from build123d import *

# Parameters (mm, degrees)
SKETCH1_R           = 1.5
SKETCH1_R_2         = 11.43
BOSS_EXTRUDE1_DEPTH = 7.62
CUT_EXTRUDE1_DEPTH  = 5.08
BOSS_EXTRUDE2_DEPTH = 2.54
SKETCH4_R           = 1
CUT_EXTRUDE2_DEPTH  = 8.62


with BuildPart() as part:
    # Sketch1 → Boss-Extrude1 (new body)
    with BuildSketch(Plane(origin=(0, 0, 0), x_dir=(1, 0, 0), z_dir=(0, 1, 0))):
        with BuildLine():
            Line((6.35, 0), (44.45, 0))
            ThreePointArc((44.45, 0), (48.940128061, 1.859871939), (50.8, 6.35))
            Line((50.8, 6.35), (50.8, 44.45))
            ThreePointArc((50.8, 44.45), (48.940128061, 48.940128061), (44.45, 50.8))
            Line((44.45, 50.8), (6.35, 50.8))
            ThreePointArc((6.35, 50.8), (1.859871939, 48.940128061), (0, 44.45))
            Line((0, 44.45), (0, 6.35))
            ThreePointArc((0, 6.35), (1.859871939, 1.859871939), (6.35, 0))
        make_face()
        with Locations((6.35, 6.35)):
            Circle(SKETCH1_R, mode=Mode.SUBTRACT)
        with Locations((6.35, 44.45)):
            Circle(SKETCH1_R, mode=Mode.SUBTRACT)
        with Locations((44.45, 44.45)):
            Circle(SKETCH1_R, mode=Mode.SUBTRACT)
        with Locations((44.45, 6.35)):
            Circle(SKETCH1_R, mode=Mode.SUBTRACT)
        with Locations((25.4, 25.4)):
            Circle(SKETCH1_R_2, mode=Mode.SUBTRACT)
    extrude(amount=BOSS_EXTRUDE1_DEPTH)

    # Sketch2 → Cut-Extrude1 (cut)
    with BuildSketch(Plane.XZ):
        with BuildLine():
            Line((8.938918626, -26.67), (0, -26.67))
            Line((0, -26.67), (0, -50.8))
            Line((0, -50.8), (24.13, -50.8))
            Line((24.13, -50.8), (24.13, -41.861081374))
            ThreePointArc((24.13, -41.861081374), (13.725667043, -37.074332957), (8.938918626, -26.67))
        make_face()
        with BuildLine():
            Line((0, 0), (0, -24.13))
            Line((0, -24.13), (8.938918626, -24.13))
            ThreePointArc((8.938918626, -24.13), (13.725667043, -13.725667043), (24.13, -8.938918626))
            Line((24.13, -8.938918626), (24.13, 0))
            Line((24.13, 0), (0, 0))
        make_face()
        with BuildLine():
            ThreePointArc((41.861081374, -26.67), (37.074332957, -37.074332957), (26.67, -41.861081374))
            Line((26.67, -41.861081374), (26.67, -50.8))
            Line((26.67, -50.8), (50.8, -50.8))
            Line((50.8, -50.8), (50.8, -26.67))
            Line((50.8, -26.67), (41.861081374, -26.67))
        make_face()
        with BuildLine():
            Line((26.67, 0), (26.67, -8.938918626))
            ThreePointArc((26.67, -8.938918626), (37.074332957, -13.725667043), (41.861081374, -24.13))
            Line((41.861081374, -24.13), (50.8, -24.13))
            Line((50.8, -24.13), (50.8, 0))
            Line((50.8, 0), (26.67, 0))
        make_face()
    extrude(amount=-CUT_EXTRUDE1_DEPTH, mode=Mode.SUBTRACT)

    # Sketch3 → Boss-Extrude2 (add)
    with BuildSketch(Plane(origin=(0, 7.62, 0), x_dir=(1, 0, 0), z_dir=(0, 1, 0))):
        with BuildLine():
            Line((35.63906734, 20.32), (15.16093266, 20.32))
            ThreePointArc((15.16093266, 20.32), (25.4, 13.97), (35.63906734, 20.32))
        make_face()
        with BuildLine():
            ThreePointArc((15.16093266, 30.48), (13.97, 25.4), (15.16093266, 20.32))
            Line((15.16093266, 20.32), (15.16093266, 30.48))
        make_face()
        with BuildLine():
            ThreePointArc((35.63906734, 30.48), (25.4, 36.83), (15.16093266, 30.48))
            Line((15.16093266, 30.48), (35.63906734, 30.48))
        make_face()
        with BuildLine():
            Line((35.63906734, 30.48), (35.63906734, 20.32))
            ThreePointArc((35.63906734, 20.32), (36.528284677, 22.791134317), (36.83, 25.4))
            ThreePointArc((36.83, 25.4), (36.528284677, 28.008865683), (35.63906734, 30.48))
        make_face()
    extrude(amount=-BOSS_EXTRUDE2_DEPTH)

    # Sketch4 → Cut-Extrude2 (cut, through all)
    with BuildSketch(Plane(origin=(0, 7.62, 0), x_dir=(1, 0, 0), z_dir=(0, 1, 0))):
        with Locations((20.24093266, 36.83)):
            Circle(SKETCH4_R)
        with Locations((32.74093266, 36.83)):
            Circle(SKETCH4_R)
        with Locations((20.24093266, 15.83)):
            Circle(SKETCH4_R)
        with Locations((32.74093266, 15.83)):
            Circle(SKETCH4_R)
    extrude(amount=-CUT_EXTRUDE2_DEPTH, mode=Mode.SUBTRACT)


solid = part.part
Geometry check sheet. Reference: the model listing, model coordinates, mm. A direction names the side the tool comes from. Round coordinates to 2 decimals unless told otherwise and drop trailing zeros. Order: outer loops, then holes, each group sorted by start corner. A loop starts at its lowest first (then second) coordinate and runs counter-clockwise, first axis right, second up. Notation, with made-up numbers: M 31,9 L 64,9 A28 ccw 64,46 Z; hole C 84.25,74 d11. An arc over 180 degrees is marked long. Answer in a Markdown table with one row per item. Add a question column.
Item 1: Draft check along X on faces 4 (the face through (24.13, 3, -46)), 5 (the face through (15, 5.08, -25)), 6 (the face through (5, 3, -26.67)). Enter one of: released by +X, released by -X, zero draft, split by the parting line, or undercut.
Item 2: Sectioned sample at A-A, the plane x = 20. Enter the section's corners in (y, z), plus the area to 3 significant figures.
Item 3: Sectioned sample at C-C, the plane x = 28. Enter the section's corners in (y, z).
Item 4: Set-up check for faces 1 (the face through (37.19, 2.5, -36.96)), 2 (the face through (26, 6, -20.32)), 3 (the face through (26.28, 2.504, -14.004)): record each of +Z, -Z, +X, -X, +Y, -Y from which the full face is reachable in a straight line by a thin tool's end or side.
Item 5: Sectioned sample at B-B, the plane z = -4. Enter the section's corners in (x, y).
Item 6: Sectioned sample at D-D, the plane y = 2.75. Enter the section's corners in (x, z), plus the area to 3 significant figures.
Item 7: Material ranges on L1, parallel to Z at x = 44.45, y = 6.85; L2, parallel to X at y = 6.3, z = -44.45; L3, parallel to Z at x = 18, y = 5.5, recorded low to high. Write a range as [from, to].
Item 8: Depth check by flat-ended pin: pin 1 Ø3 at (y, z) = (2.5, -16.5) entering from +X; pin 2 Ø3 at (x, z) = (23.5, -18.5) entering from -Y; pin 3 Ø1.5 at (x, y) = (13, 3) entering from +Z. Enter the tip coordinate at first touch or a pass-through.
Filled in:
| question | item | result |
|---|---|---|
| 1 | face 4 | released by -X |
| 1 | face 5 | undercut |
| 1 | face 6 | zero draft |
| 2 | outline | M 0,-41 L 5.08,-41 L 5.08,-50.8 L 7.62,-50.8 L 7.62,-37.8 L 0,-37.8 Z; M 0,-35.86 L 7.62,-35.86 L 7.62,-30.48 L 5.08,-30.48 L 5.08,-35.47 L 0,-35.47 Z; M 0,-14.86 L 7.62,-14.86 L 7.62,0 L 5.08,0 L 5.08,-9.8 L 0,-9.8 Z; M 5.08,-20.32 L 7.62,-20.32 L 7.62,-16.8 L 5.08,-16.8 Z |
| 2 | area | 137 mm² |
| 3 | outline | M 0,-41.7 L 5.08,-41.7 L 5.08,-50.8 L 7.62,-50.8 L 7.62,-30.48 L 5.08,-30.48 L 5.08,-36.53 L 0,-36.53 Z; M 0,-14.27 L 5.08,-14.27 L 5.08,-20.32 L 7.62,-20.32 L 7.62,0 L 5.08,0 L 5.08,-9.1 L 0,-9.1 Z |
| 4 | face 1 | -Z, +X, -Y |
| 4 | face 2 | +Y, -Y |
| 4 | face 3 | -Y |
| 5 | outline | M 0.45,5.08 L 24.13,5.08 L 24.13,0 L 26.67,0 L 26.67,5.08 L 50.35,5.08 L 50.35,7.62 L 0.45,7.62 Z |
| 6 | outline | M 0,-26.67 L 8.94,-26.67 A16.51 ccw 24.13,-41.86 L 24.13,-50.8 L 26.67,-50.8 L 26.67,-41.86 A16.51 ccw 41.86,-26.67 L 50.8,-26.67 L 50.8,-24.13 L 41.86,-24.13 A16.51 ccw 26.67,-8.94 L 26.67,0 L 24.13,0 L 24.13,-8.94 A16.51 ccw 8.94,-24.13 L 0,-24.13 Z; hole C 20.24,-36.83 d2; hole M 19.24,-15.77 A11.43 ccw long 32.94,-16.81 A1 ccw long 31.74,-15.89 A11.43 ccw 20.74,-14.96 A1 ccw Z; hole C 32.74,-36.83 d2 |
| 6 | area | 527 mm² |
| 7 | L1 | z = [-50.8, -45.95], [-42.95, -7.85], [-4.85, 0] |
| 7 | L2 | x = [0, 4.85], [7.85, 42.95], [45.95, 50.8] |
| 7 | L3 | z = [-50.8, -30.48], [-20.32, 0] |
| 8 | pin 1 | stops at x = 40.16 |
| 8 | pin 2 | stops at y = 5.08 |
| 8 | pin 3 | stops at z = -13.7 |
